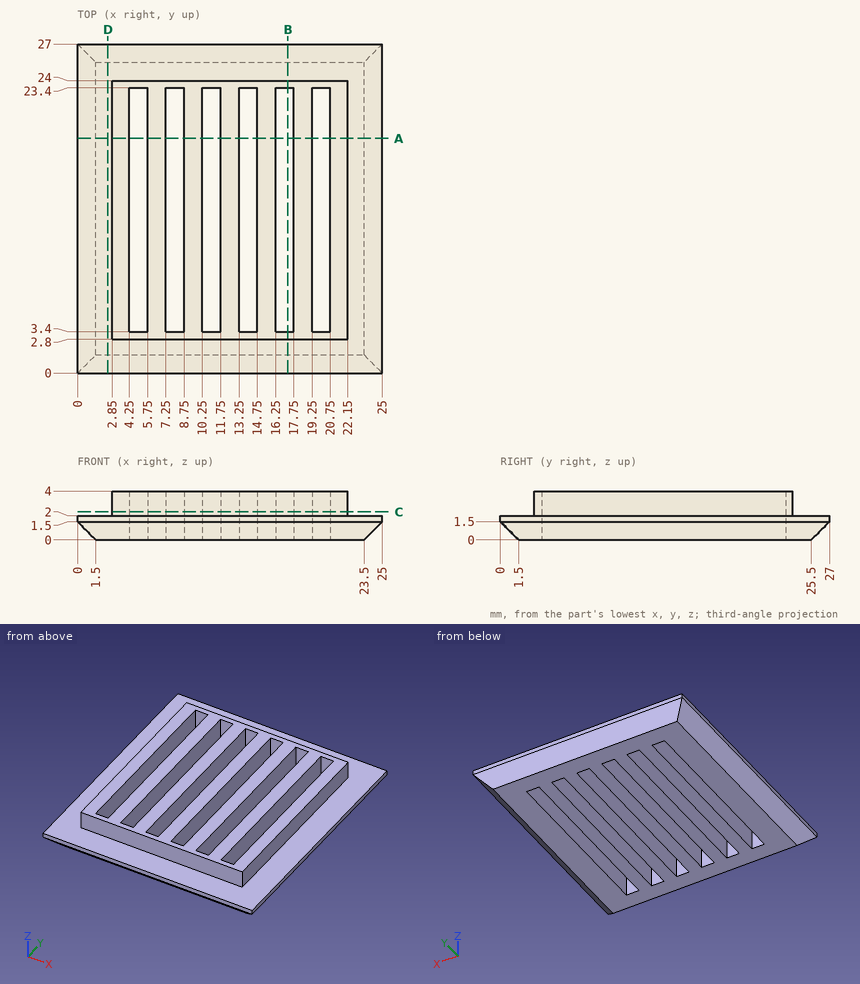
Study the drawing (mm; zero at the part's minimum x, y, z) and answer. Give positions to 0.01 mm unless a question says otherwise; leave off trailing zeros. Loops run counter-clockwise (first coordinate to the right, second up) from the corner with the lowest first, then second, coordinate; pieces in that order, holes last. Notation, with made-up numbers: M -18,31 L 12,31 A21 cw 12,52 Z; hole C -33.75,5 d3. An arc over 180 degrees is marked long. Answer as CSV lines item,"result".
Item 1: Straight lines are drawn through the part: line 1 along Y through (x, z) = (13.5, 1.7); line 2 along Z through (x, y) = (13, 1.75); line 3 along Y through (x, z) = (3, 2.35). For each, find the intervals that lie inside material, in ascending order. Write a range as [from, to].
Values follow:
line 1,"y = [0, 3.4], [23.4, 27]"
line 2,"z = [0, 2]"
line 3,"y = [2.8, 24]"
Item 2: The part is cut by section B-B (x = 17.25). Give the vertices of the cut face in (y, z), and give its area (4 significant figures).
Values follow:
outline,"M 0,1.5 L 1.5,0 L 3.4,0 L 3.4,4 L 2.8,4 L 2.8,2 L 0,2 Z; M 23.4,0 L 25.5,0 L 27,1.5 L 27,2 L 24,2 L 24,4 L 23.4,4 Z"
area,"14.15 mm^2"
Item 3: The part is cut by section A-A (y = 19.25). Give the number of separate pieces and of enclosed holes in the cut face, and give its area (4 significant figures).
Values follow:
separate pieces,"7"
enclosed holes,"0"
area,"50.35 mm^2"
Item 4: The part is cut by section C-C (z = 2.3). Give the vertices of the cut face in (x, y), and give its area (3 significant figures).
Values follow:
outline,"M 2.85,2.8 L 22.15,2.8 L 22.15,24 L 2.85,24 Z; hole M 4.25,3.4 L 5.75,3.4 L 5.75,23.4 L 4.25,23.4 Z; hole M 7.25,3.4 L 8.75,3.4 L 8.75,23.4 L 7.25,23.4 Z; hole M 10.25,3.4 L 11.75,3.4 L 11.75,23.4 L 10.25,23.4 Z; hole M 13.25,3.4 L 14.75,3.4 L 14.75,23.4 L 13.25,23.4 Z; hole M 16.25,3.4 L 17.75,3.4 L 17.75,23.4 L 16.25,23.4 Z; hole M 19.25,3.4 L 20.75,3.4 L 20.75,23.4 L 19.25,23.4 Z"
area,"229 mm^2"
Item 5: The part is cut by section D-D (x = 2.5). Give the vertices of the cut face in (y, z).
Values follow:
outline,"M 0,1.5 L 1.5,0 L 25.5,0 L 27,1.5 L 27,2 L 0,2 Z"
Item 6: Given pin 1 Ø1.6 at (y, z) = (16, 3) entering from +X; pin 2 Ø1.6 at (x, z) = (14, 3) entering from -Y; pin 3 Ø1 at (x, z) = (11, 3) entering from +Y, each flat-ended and moving along its own axis, determine where each tip first touches the part or whether it passes through.
Values follow:
pin 1,"stops at x = 22.15"
pin 2,"stops at y = 2.8"
pin 3,"stops at y = 24"
